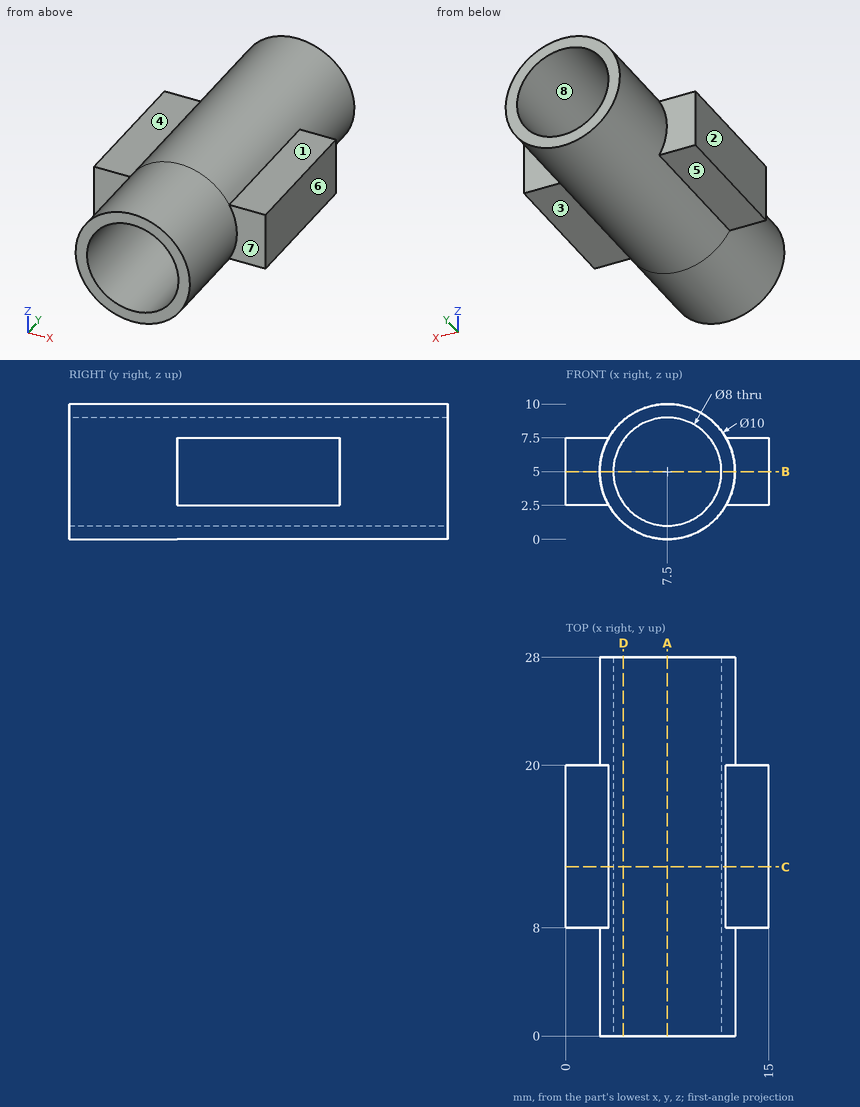
Answer from the drawing. Dimensions are ordinates in mm from the lowest x, y and z of the part. A direction names the side the tool comes from. Give positions to 0.01 mm unless a question says otherwise; leave off trailing zeros. Order: outer loops, then holes, each group sorted by start corner. A loop starts at its lowest first (then second) coordinate and runs counter-clockwise, first axis right, second up. Notation, with made-up numbers: (75, 71.25) -> (132, 71.25) arc R17 cw to (132, 104.25) -> close; hole circle Ø6 at (80.5, 24). An arc over 180 degrees is marked (long way). Answer as a JSON object with one key per item and string values. Group by question number.
1. Flat-ended cylindrical pins translate along their axes: pin 1 Ø1 at (x, z) = (13.5, 6) entering from -Y; pin 2 Ø2.5 at (x, y) = (13.5, 11) entering from +Z; pin 3 Ø3 at (x, y) = (3.5, 19.5) entering from +Z; pin 4 Ø2 at (x, z) = (9, 2.5) entering from +Y. Find the tip coordinate at first contact, or state that the pin passes through.
2. Section D-D on x = 4.25 is taken. Determine the outline of the cut face in (y, z).
3. Consider line 1 along X through (y, z) = (3.75, 5); line 2 along X through (y, z) = (8.75, 5); line 3 along Z through (x, y) = (5.75, 20.5). Determine where each line is inside the solid, lowest interval first. Write a range as [from, to].
4. Section A-A on x = 7.5 is taken. Determine the outline of the cut face in (y, z), plus the area to 3 significant figures.
5. The mould has two halves that part along X. Classify the marked faces 6, 7 and 8: released by +X, released by -X, zero draft, split by the parting line, or undercut.
6. Section C-C on y = 12.5 is taken. Determine the outline of the cut face in (x, z), plus the area to 3 significant figures.
7. Section B-B on z = 5 is taken. Determine the outline of the cut face in (x, y), plus the area to 3 significant figures.
8. A tool of negligible diameter and unlimited length cuts with its end or side. For the marked faces 1, 2, 3, 4 and 5, from which of +Z, -Z, +X, -X, +Y, -Y can it reach the whole face along a straight path? Write none if from no direction.
Result sheet:
{
 "1": {"pin 1": "stops at y = 8", "pin 2": "stops at z = 7.5", "pin 3": "stops at z = 9.33", "pin 4": "passes through"},
 "2": {"outline": "(0, 1.2) -> (28, 1.2) -> (28, 2.67) -> (0, 2.67) -> close; (0, 7.33) -> (28, 7.33) -> (28, 8.8) -> (0, 8.8) -> close"},
 "3": {"line 1": "x = [2.5, 3.5], [11.5, 12.5]", "line 2": "x = [0, 3.5], [11.5, 15]", "line 3": "z = [0.32, 1.4], [8.6, 9.68]"},
 "4": {"outline": "(0, 0) -> (28, 0) -> (28, 1) -> (0, 1) -> close; (0, 9) -> (28, 9) -> (28, 10) -> (0, 10) -> close", "area": "56.0 mm^2"},
 "5": {"face 6": "released by +X", "face 7": "zero draft", "face 8": "undercut"},
 "6": {"outline": "(0, 2.5) -> (3.17, 2.5) arc R5 ccw to (11.83, 2.5) -> (15, 2.5) -> (15, 7.5) -> (11.83, 7.5) arc R5 ccw to (3.17, 7.5) -> (0, 7.5) -> close; hole circle Ø8 at (7.5, 5)", "area": "55.4 mm^2"},
 "7": {"outline": "(0, 8) -> (2.5, 8) -> (2.5, 0) -> (3.5, 0) -> (3.5, 28) -> (2.5, 28) -> (2.5, 20) -> (0, 20) -> close; (11.5, 0) -> (12.5, 0) -> (12.5, 8) -> (15, 8) -> (15, 20) -> (12.5, 20) -> (12.5, 28) -> (11.5, 28) -> close", "area": "116 mm^2"},
 "8": {"face 1": "+Z, +X, +Y, -Y", "face 2": "+Z, -Z, -X, +Y, -Y", "face 3": "-Z, +X, +Y, -Y", "face 4": "+Z, -X, +Y, -Y", "face 5": "-Z, -X, +Y, -Y"}
}
